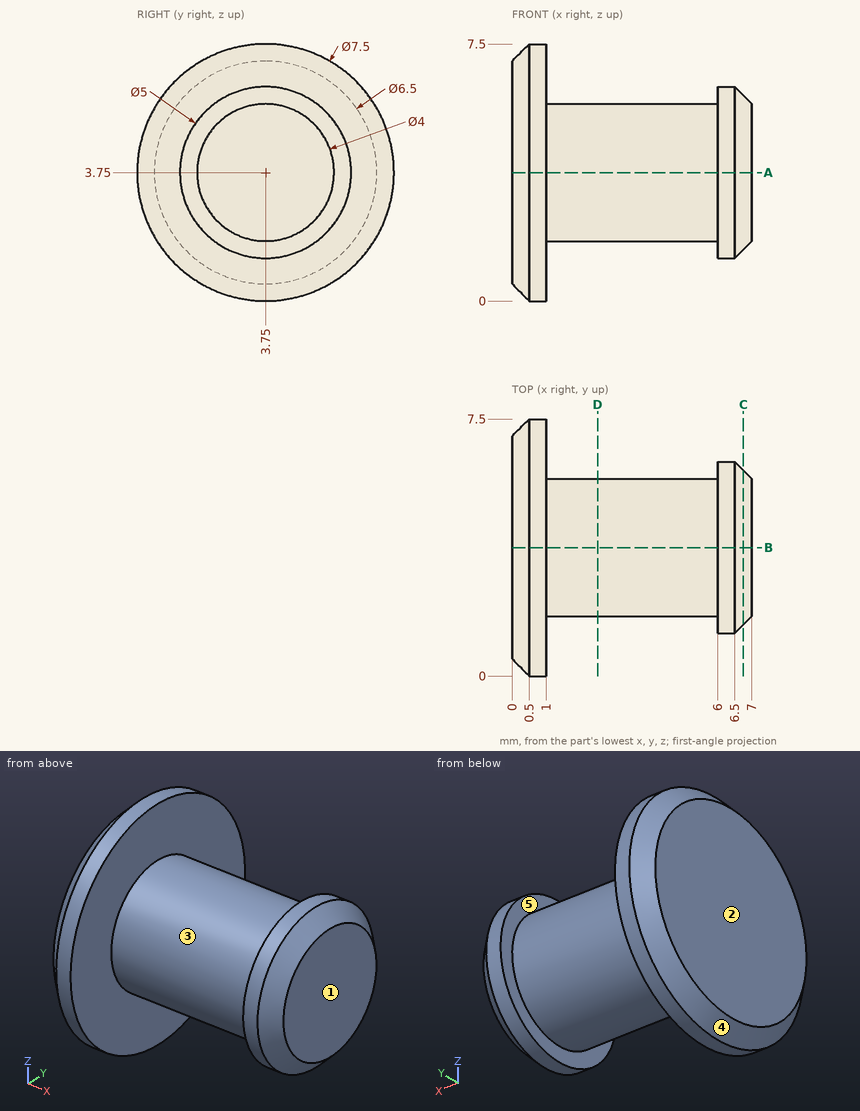
Print and shaded views of the part. All mm, measured from the part's lowest x, y and z. A direction names the side the tool comes from. Coordinates: 2 decimals unless noted, no trailing zeros. Order: outer loops, then holes, each group sorted by start corner. A loop starts at its lowest first (then second) coordinate and runs counter-clockwise, first axis right, second up.
Item 1: Mould opens along X. For the marked faces 1, 2 and 3 say: released by +X, released by -X, zero draft, split by the parting line, or undercut.
Filled in:
face 1: released by +X
face 2: released by -X
face 3: undercut
Item 2: Drop flat-ended pins along their axis: pin 1 Ø1 at (x, y) = (3, 2) entering from -Z; pin 2 Ø2 at (x, z) = (5.5, 6.5) entering from +Y; pin 3 Ø1.5 at (x, y) = (4.5, 2) entering from -Z. Give the stop position or say it passes through.
Filled in:
pin 1: stops at z = 2.19
pin 2: stops at y = 5.39
pin 3: stops at z = 2.02
Item 3: Saw through at C-C on x = 6.75. List the corners of the cut face in (y, z).
Filled in:
outline: circle Ø4.5 at (3.75, 3.75)
Item 4: Saw through at A-A on z = 3.75. List the corners of the cut face in (x, y).
Filled in:
outline: (0, 0.5) - (0.5, 0) - (1, 0) - (1, 1.75) - (6, 1.75) - (6, 1.25) - (6.5, 1.25) - (7, 1.75) - (7, 5.75) - (6.5, 6.25) - (6, 6.25) - (6, 5.75) - (1, 5.75) - (1, 7.5) - (0.5, 7.5) - (0, 7) - close
Item 5: Saw through at D-D on x = 2.5. List the corners of the cut face in (y, z), then the cut area to 3 significant figures.
Filled in:
outline: circle Ø4 at (3.75, 3.75)
area: 12.6 mm2
Item 6: Tool access for the marked faces 4 and 5: list every direction of +Z, -Z, +X, -X, +Y, -Y with a clear straight run to the whole face (end or side of a thin tool).
Filled in:
face 4: -X
face 5: none
Item 7: Drill centre lines: L1, parallel to X at y = 2.25, z = 6; L2, parallel to X at y = 5.25, z = 5.5; L3, parallel to X at y = 4.25, z = 5.75. Where is each one in solid material? Low to high.
Filled in:
L1: x = 0 to 1
L2: x = 0 to 1, 6 to 6.7
L3: x = 0 to 1, 6 to 6.94
